Part model, mm, in its own coordinate system. Face numbers are marked on the shaded views. A direction names the side the tool comes from. Give positions to 0.01 mm unless a question says otherwise; leave off trailing zeros. Order: outer loops, then holes, each group sorted by start corner. A loop starts at its lowest first (then second) coordinate and runs counter-clockwise, first axis right, second up. Notation, with made-up numbers: (-19, -21.75) -> (14, -21.75) arc R10 cw to (14, -16.75) -> close; hole circle Ø8 at (39.5, 63). An arc over 180 degrees is marked (long way). Write item = value, one per line. Start each with the question number.
Item 1: Drill centre lines: line 1 along Y through (x, z) = (127, 47); line 2 along Y through (x, z) = (243, 46); line 3 along Z through (x, y) = (251.5, 151.5) (3 decimals). Where is each one in solid material? Low to high.
Item 2: Flat gauge pins, fed straight in: P1, Ø12, axis at x = 238, z = 79, coming from the +Y side; P2, Ø4, axis at x = 98.5, y = 246.5, coming from the +Z side (3 decimals); P3, Ø1, axis at x = 57, z = 46, coming from the +Y side. Where does each tip first touch, or does it go through?
Item 3: Tool access for the marked faces 1 and 2: list every direction of +Z, -Z, +X, -X, +Y, -Y with a clear straight run to the whole face (end or side of a thin tool).
Item 4: Band-saw the part on A-A on x = 182. Write the cut outline in (y, z) (3 decimals), plus the area to 3 significant figures.
Item 5: Band-saw the part on B-B on z = 62. Write the cut outline in (x, y) (3 decimals).
Item 6: Band-saw the part on C-C on y = 102. Write the cut outline in (x, z) (3 decimals).
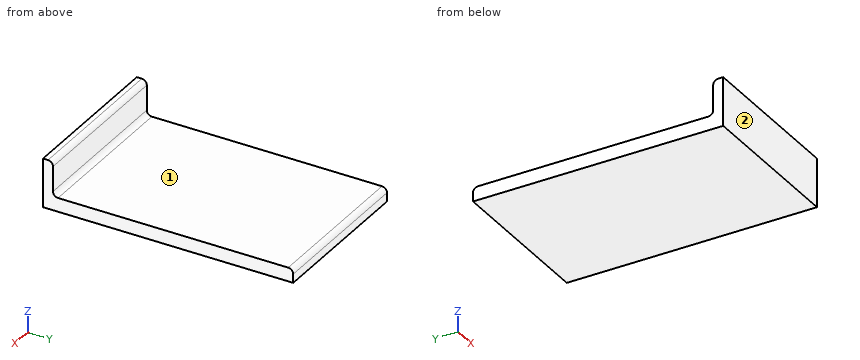
```python
from build123d import *

# Parameters (mm, degrees)
F1_DEPTH = 403.225


with BuildPart() as f1:
    # F0 (on Right) → F1 (new body)
    with BuildSketch(Plane.YZ):
        with BuildLine():
            Line((0, 123.825), (0, 0))
            Line((0, 0), (635, 0))
            Line((635, 0), (635, 22.225))
            ThreePointArc((635, 22.225), (631.280256, 31.205256), (622.3, 34.925))
            Line((622.3, 34.925), (38.1, 34.925))
            ThreePointArc((38.1, 34.925), (29.119744, 38.644744), (25.4, 47.625))
            Line((25.4, 47.625), (25.4, 111.125))
            ThreePointArc((25.4, 111.125), (21.680256, 120.105256), (12.7, 123.825))
            Line((12.7, 123.825), (0, 123.825))
        make_face()
    extrude(amount=F1_DEPTH)


solid = f1.part
```
Values found:
q1.line_1 = 0 to 25.42
q1.line_2 = 0 to 25.5
q1.line_3 = 0 to 34.925
q2.P1 = 25.4
q2.P2 = 34.925
q2.P3 = 25.58
q3.face_1 = +Z, +X, -X, +Y
q3.face_2 = +Z, -Z, +X, -X, -Y
q4.outline = (0, 0) -> (635, 0) -> (635, 22.225) arc R12.7 ccw to (622.3, 34.925) -> (38.1, 34.925) arc R12.7 cw to (25.4, 47.625) -> (25.4, 111.125) arc R12.7 ccw to (12.7, 123.825) -> (0, 123.825) -> close
q4.area = 24,400 mm^2
q5.outline = (0, 0) -> (403.225, 0) -> (403.225, 25.4) -> (0, 25.4) -> close
q6.outline = (0, 0) -> (403.225, 0) -> (403.225, 34.925) -> (0, 34.925) -> close
